For this review, take the finished solid that the model builds, in its own axes (mm). A direction names the side the tool comes from. Coordinates: 2 decimals unless noted, no trailing zeros. Order: outer loops, then holes, each group sorted by start corner. A loop starts at its lowest first (then second) coordinate and runs counter-clockwise, first axis right, second up. Notation, with made-up numbers: (72.25, 2.25) -> (89.25, 2.25) arc R32 ccw to (89.25, 41.25) -> close; hole circle Ø5 at (45.25, 55.25). An arc over 180 degrees is marked (long way). Write item = value, one per line. Start each with the question number.
1) Machinability: for faces 5 (the face through (-56, 23, 1.55)), 6 (the face through (-1, 35, 16)), 7 (the face through (-50.225, -8.784, 42.62)), 8 (the face through (0, 0, 5)), which of the approach directions +Z, -Z, +X, -X, +Y, -Y give a long, thin tool a straight path to every point of the face, cutting with its end or side? Answer none if there is none.
2) Consider section C-C on x = 22. Give the boundary of the cut face in (y, z).
3) Wall thickness on probe 1 along Y at (x, z) = (0, -2.5); probe 2 along Z at (x, y) = (32, 8.5); probe 3 along X at (y, z) = (26, 4): over which ranges is each line inside the solid? List them lowest first. Write a range as [from, to].
4) Draft analysis for pull direction Z (two halves, no side actions). For faces 1 (the face through (31, -33, 23)), 2 (the face through (-30, 0, 40.155)), 3 (the face through (-56, 23, -2.42)), 4 (the face through (-62.5, -6, 31)), state which applies: +Z half, -Z half, draft (parallel to the pull), parting line (faces both ways), or undercut.
5) Consider section B-B on z = 27. Give the boundary of the cut face in (x, y).
6) Insertion check: pin 1 Ø2 at (y, z) = (21.5, 7) entering from -X; pin 2 Ø6 at (y, z) = (-12.5, 38) entering from -X; pin 3 Ø4 at (x, y) = (-19.5, -18) entering from +Z. Each pin has a flat end and moves straight along its axis. Give the tip position at first contact, or say it passes through.
7) Consider section D-D on y = 15.5. Give the boundary of the cut face in (x, z), and give its area (3 significant figures).
8) Consider section A-A on y = 24. Give the boundary of the cut face in (x, z), and give its area (3 significant figures).
from build123d import *

# Parameters (mm, degrees)
SKETCH4_W                = 120
SKETCH4_H                = 70
BOSS_EXTRUDE1_DEPTH      = 10
SKETCH5_R                = 5
CUT_EXTRUDE1_DEPTH       = 40
BOSS_EXTRUDE2_DEPTH      = 70
SKETCH9_R                = 5
CUT_EXTRUDE2_DEPTH       = 15
SKETCH11_R               = 25
BOSS_EXTRUDE3_DEPTH      = 5
BOSS_EXTRUDE3_DEPTH_BACK = 10
SKETCH12_R               = 5
CUT_EXTRUDE3_DEPTH       = 7
BOSS_EXTRUDE5_DEPTH      = 5
SKETCH15_W               = 4.5
SKETCH15_H               = 10
CUT_EXTRUDE4_DEPTH       = 8
SKETCH16_W               = 1.569022944
SKETCH16_H               = 8.700945414
SKETCH16_W_2             = 1.426384494
BOSS_EXTRUDE6_DEPTH      = 8
SKETCH17_W               = 40.700182708
SKETCH17_H               = 28.264015769
BOSS_EXTRUDE7_DEPTH      = 1
BOSS_EXTRUDE8_DEPTH      = 1.5


with BuildPart() as part:
    # Sketch4 → Boss-Extrude1 (new body)
    with BuildSketch(Plane.XY):
        Rectangle(SKETCH4_W, SKETCH4_H)
    extrude(amount=-BOSS_EXTRUDE1_DEPTH)

    # Sketch5 → Cut-Extrude1 (cut)
    with BuildSketch(Plane.XY):
        Circle(SKETCH5_R)
    extrude(amount=-CUT_EXTRUDE1_DEPTH, mode=Mode.SUBTRACT)

    # Sketch8 → Boss-Extrude2 (add)
    with BuildSketch(Plane.XZ.offset(35)):
        with BuildLine():
            Line((-60, -10), (-60, 40.154750478))
            Line((-60, 40.154750478), (0, 40.154750478))
            ThreePointArc((0, 40.154750478), (33.3625471, 35.597841439), (60, 15))
            Line((60, 15), (60, -10))
            Line((60, -10), (-60, -10))
        make_face()
    extrude(amount=-BOSS_EXTRUDE2_DEPTH)

    # Sketch9 → Cut-Extrude2 (cut)
    with BuildSketch(Plane(origin=(0, 0, -10), x_dir=(-1, 0, 0), z_dir=(0, 0, -1))):
        Circle(SKETCH9_R)
    extrude(amount=-CUT_EXTRUDE2_DEPTH, mode=Mode.SUBTRACT)

    # Sketch11 → Boss-Extrude3 (add, two sides)
    with BuildSketch(Plane.XZ.offset(35)) as boss_extrude3_sk:
        with Locations((31.117439105, 23.306323577)):
            Circle(SKETCH11_R)
    extrude(amount=BOSS_EXTRUDE3_DEPTH)
    extrude(boss_extrude3_sk.sketch, amount=-BOSS_EXTRUDE3_DEPTH_BACK)

    # Sketch12 → Cut-Extrude3 (cut)
    with BuildSketch(Plane.XZ.offset(40)):
        with Locations((31.117439105, 23.306323577)):
            Circle(SKETCH12_R)
    extrude(amount=-CUT_EXTRUDE3_DEPTH, mode=Mode.SUBTRACT)

    # Sketch14 → Boss-Extrude5 (add)
    with BuildSketch(Plane.XY.offset(40.154750478)):
        with BuildLine():
            Line((-45.98826123, -12.928324025), (-45.98826123, -24.846408626))
            ThreePointArc((-45.98826123, -24.846408626), (-50.13368196, -28.991829356), (-54.279102691, -24.846408626))
            Line((-54.279102691, -24.846408626), (-54.279102691, -12.928324025))
            ThreePointArc((-54.279102691, -12.928324025), (-50.13368196, -8.782903295), (-45.98826123, -12.928324025))
        make_face()
    extrude(amount=BOSS_EXTRUDE5_DEPTH)

    # Sketch15 → Cut-Extrude4 (cut)
    with BuildSketch(Plane.ZY.offset(60)):
        with Locations((-0.699635799, 23.193765021)):
            Rectangle(SKETCH15_W, SKETCH15_H)
        with Locations((6.524606685, 23.193765021)):
            Rectangle(SKETCH15_W, SKETCH15_H)
    extrude(amount=-CUT_EXTRUDE4_DEPTH, mode=Mode.SUBTRACT)

    # Sketch16 → Boss-Extrude6 (add)
    with BuildSketch(Plane.ZY.offset(52)):
        with Locations((-1.63562366, 23.437743986)):
            Rectangle(SKETCH16_W, SKETCH16_H)
        with Locations((5.710256485, 23.437743986)):
            Rectangle(SKETCH16_W_2, SKETCH16_H)
    extrude(amount=BOSS_EXTRUDE6_DEPTH)

    # Sketch17 → Boss-Extrude7 (add)
    with BuildSketch(Plane.ZY.offset(60)):
        with Locations((16.084407409, -14.726216905)):
            Rectangle(SKETCH17_W, SKETCH17_H)
    extrude(amount=BOSS_EXTRUDE7_DEPTH)

    # Sketch18 → Boss-Extrude8 (add)
    with BuildSketch(Plane.ZY.offset(61)):
        Polygon((-0.506912877, -8.264193133), (2.379724675, -8.289824612), (3.845240963, -5.802738899), (2.424119698, -3.290021707), (-0.462517855, -3.264390229), (-1.928034142, -5.751475942), align=None)
        Polygon((34.09684896, -5.751475942), (32.675727695, -8.264193133), (29.789090142, -8.289824612), (28.323573855, -5.802738899), (29.74469512, -3.290021707), (32.631332673, -3.264390229), align=None)
        Polygon((-1.928034142, -23.700957867), (-0.506912877, -21.188240676), (2.379724675, -21.162609198), (3.845240963, -23.649694911), (2.424119698, -26.162412102), (-0.462517855, -26.18804358), align=None)
        Polygon((32.675727695, -21.188240676), (29.789090142, -21.162609198), (28.323573855, -23.649694911), (29.74469512, -26.162412102), (32.631332673, -26.18804358), (34.09684896, -23.700957867), align=None)
    extrude(amount=BOSS_EXTRUDE8_DEPTH)


solid = part.part
Answer sheet:
q1.face_5 = -X
q1.face_6 = +Z, -Z, +X, -X, +Y
q1.face_7 = +Z, +Y
q1.face_8 = -Z
q2.outline = (-40, 0.03) -> (-35, 0.03) -> (-35, -10) -> (35, -10) -> (35, 39.18) -> (-25, 39.18) -> (-25, 46.58) -> (-40, 46.58) -> close
q3.probe_1 = [-35, -5], [5, 35]
q3.probe_2 = [-10, 36.15]
q3.probe_3 = [-60, 60]
q4.face_1 = undercut
q4.face_2 = +Z half
q4.face_3 = undercut
q4.face_4 = draft
q5.outline = (-61, -28.86) -> (-60, -28.86) -> (-60, -35) -> (6.39, -35) -> (6.39, -40) -> (27.75, -40) -> (27.75, -33) -> (34.49, -33) -> (34.49, -40) -> (55.84, -40) -> (55.84, -25) -> (48.1, -25) -> (48.1, 35) -> (-60, 35) -> (-60, -0.59) -> (-61, -0.59) -> close
q6.pin_1 = -60
q6.pin_2 = -61
q6.pin_3 = 40.15
q7.outline = (-60, -10) -> (60, -10) -> (60, 15) arc R65.19 ccw to (0, 40.15) -> (-60, 40.15) -> close
q7.area = 5,650 mm2
q8.outline = (-60, -10) -> (60, -10) -> (60, 15) arc R65.19 ccw to (0, 40.15) -> (-60, 40.15) -> (-60, 8.77) -> (-52, 8.77) -> (-52, 6.42) -> (-60, 6.42) -> (-60, 5) -> (-52, 5) -> (-52, 4.27) -> (-60, 4.27) -> (-60, 1.55) -> (-52, 1.55) -> (-52, -0.85) -> (-60, -0.85) -> (-60, -2.42) -> (-52, -2.42) -> (-52, -2.95) -> (-60, -2.95) -> close
q8.area = 5,600 mm2
